Verification items for the finished model (mm, model axes). Coordinates: 2 decimals unless noted, no trailing zeros. Write each loop counter-clockwise with the first axis right and the second up, starting at its lowest first coordinate (ties: lowest second). Pieces come first, ordered by that corner, then holes. Notation, with made-up numbers: (67.5, 87) -> (115.5, 87) arc R29 ccw to (115.5, 119) -> close; hole circle Ø11 at (-29, 63). An arc over 180 degrees is marked (long way). Write each question's results on one line, items separated by ' | '. Start each with the question number.
from build123d import *

# Parameters (mm, degrees)
ESQUISSE1_W             = 120
ESQUISSE1_H             = 30
BOSS_EXTRU_1_DEPTH      = 5
ESQUISSE2_R             = 8
ESQUISSE2_R_2           = 5
ENL_V_MAT_EXTRU_1_DEPTH = 10
CONG_1_R                = 10


with BuildPart() as part:
    # Esquisse1 → Boss.-Extru.1 (new body)
    with BuildSketch(Plane.XY):
        Rectangle(ESQUISSE1_W, ESQUISSE1_H)
    extrude(amount=BOSS_EXTRU_1_DEPTH)

    # Esquisse2 → Enlèv. mat.-Extru.1 (cut)
    with BuildSketch(Plane.XY.offset(5)):
        with Locations((-44, 0)):
            Circle(ESQUISSE2_R)
        with Locations((44, 0)):
            Circle(ESQUISSE2_R_2)
    extrude(amount=-ENL_V_MAT_EXTRU_1_DEPTH, mode=Mode.SUBTRACT)

    # Congé1
    cong_1_edges = [part.edges().sort_by_distance(p)[0] for p in [
        (-60, 15, 2.5),
        (60, 15, 2.5),
        (60, -15, 2.5),
        (-60, -15, 2.5),
    ]]
    fillet(cong_1_edges, radius=CONG_1_R)


solid = part.part
1. Sectioned sample at C-C on z = 2.3. Record the cut outline in (x, y), plus the area to 3 significant figures.
2. Sectioned sample at B-B on x = 44. Record the cut outline in (y, z).
3. Material ranges on probe 1 along Y at (x, z) = (-44, 3.05); probe 2 along Y at (x, z) = (44, 3.1); probe 3 along X at (y, z) = (-1, 0.45), recorded low to high. Write a range as from..to.
4. Depth check by flat-ended pin: pin 1 Ø13 at (x, y) = (-44, 0) entering from -Z; pin 2 Ø2 at (y, z) = (7.5, 4.5) entering from -X. Enter the tip coordinate at first touch or a pass-through.
5. Sectioned sample at D-D on y = -6.5. Record the cut outline in (x, z), plus the area to 3 significant figures.
6. Sectioned sample at A-A on y = 0. Record the cut outline in (x, z), plus the area to 3 significant figures.
7. Mould release check, pull along X, two halves, no side actions. Record for faces 1 (the cylindrical face through (-57.15, -11.99, 2.54)), 2 (the cylindrical face through (-50.349, -4.868, 2.535)), 3 (the flat face through (-1, -15, 2)), 4 (the cylindrical face through (56.99, -12.15, 2.54)): +X half, -X half, draft (parallel to the pull), parting line (faces both ways), or undercut.
Computed values:
1) outline: (-60, -5) arc R10 ccw to (-50, -15) -> (50, -15) arc R10 ccw to (60, -5) -> (60, 5) arc R10 ccw to (50, 15) -> (-50, 15) arc R10 ccw to (-60, 5) -> close; hole circle Ø16 at (-44, 0); hole circle Ø10 at (44, 0) | area: 3,230 mm^2
2) outline: (-15, 0) -> (-5, 0) -> (-5, 5) -> (-15, 5) -> close; (5, 0) -> (15, 0) -> (15, 5) -> (5, 5) -> close
3) probe 1: y = -15..-8, 8..15 | probe 2: y = -15..-5, 5..15 | probe 3: x = -60..-51.94, -36.06..39.1, 48.9..60
4) pin 1: passes through | pin 2: stops at x = -59.89
5) outline: (-59.89, 0) -> (-48.66, 0) -> (-48.66, 5) -> (-59.89, 5) -> close; (-39.34, 0) -> (59.89, 0) -> (59.89, 5) -> (-39.34, 5) -> close | area: 552 mm^2
6) outline: (-60, 0) -> (-52, 0) -> (-52, 5) -> (-60, 5) -> close; (-36, 0) -> (39, 0) -> (39, 5) -> (-36, 5) -> close; (49, 0) -> (60, 0) -> (60, 5) -> (49, 5) -> close | area: 470 mm^2
7) face 1: -X half | face 2: undercut | face 3: draft | face 4: +X half
